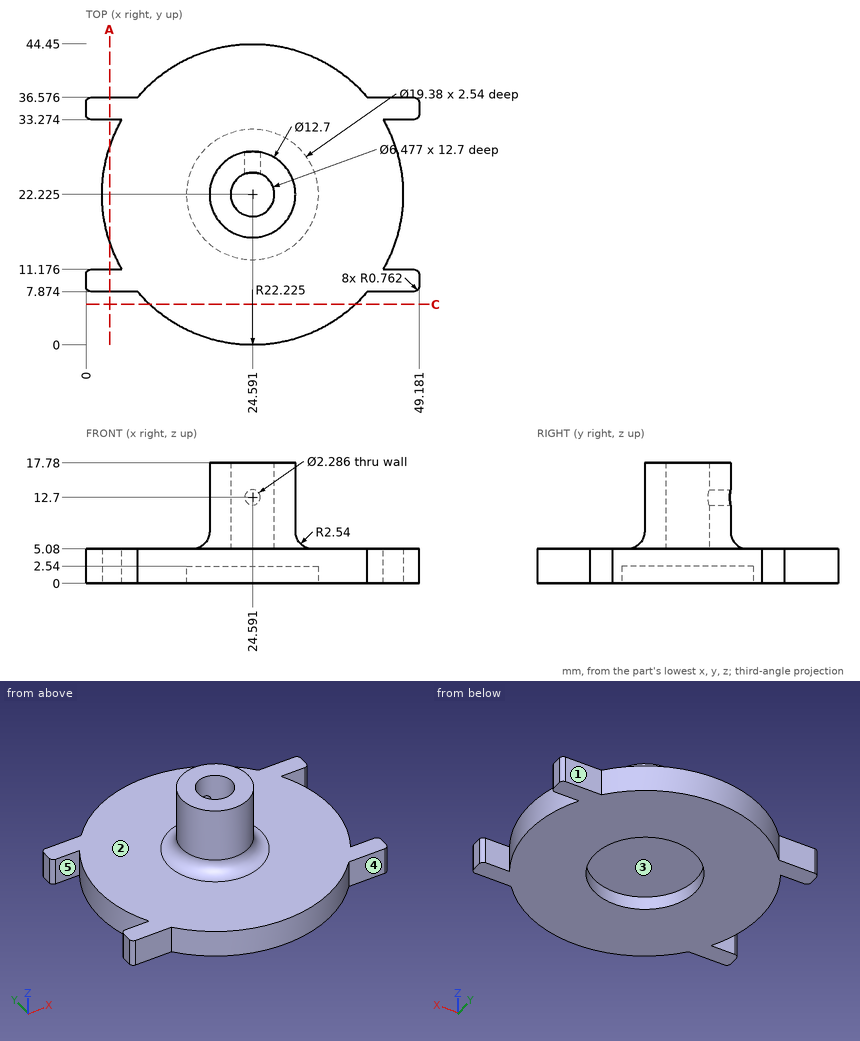
Print and shaded views of the part. All mm, measured from the part's lowest x, y and z. A direction names the side the tool comes from. Give positions to 0.01 mm unless a question says otherwise; leave off trailing zeros. Write each loop counter-clockwise with the first axis right and the second up, starting at its lowest first coordinate (ties: lowest second). Pieces come first, ordered by that corner, then holes. Notation, with made-up numbers: (63.5, 35.5) -> (110.5, 35.5) arc R35 cw to (110.5, 70.5) -> close; hole circle Ø1 at (41.5, 55.5). An arc over 180 degrees is marked (long way). Use CSV: the item, a comma, the result in double quotes. Start each with the question number.
1) Drill centre lines: L1, parallel to Z at x = 13, y = 14; L2, parallel to Y at x = 26.5, z = 7.5 (1 decimal); L3, parallel to X at y = 25, z = 12.75 (1 decimal). Where is each one in solid material? Low to high.
2) Cut at C-C on y = 6. List the corners of the cut face in (x, z).
3) Cut at A-A on x = 3.5. List the corners of the cut face in (y, z) (1 decimal), plus the area to 3 significant figures.
4) Tool access for the marked faces 1, 2, 3, 4 and 5: list every direction of +Z, -Z, +X, -X, +Y, -Y with a clear straight run to the whole face (end or side of a thin tool).
5) Pin check, flat tips, straight feed: P1, Ø5.5, axis at x = 43.5, z = 3, coming from the +Y side (1 decimal); P2, Ø3, axis at x = 25.5, y = 21.5, coming from the +Z side; P3, Ø2.5, axis at x = 3, z = 3.5, coming from the +Y side; P4, Ø10, axis at y = 8, z = 14.5, coming from the +X side. Stop position of each tip, or through.
Final values:
1,L1,"z = 0 to 5.08"
1,L2,"y = 16.2 to 19.6, 24.8 to 28.3"
1,L3,"x = 18.9 to 22.9, 26.3 to 30.3"
2,outline,"(9.4, 0) -> (39.78, 0) -> (39.78, 5.08) -> (9.4, 5.08) -> close"
3,outline,"(7.9, 0) -> (11.2, 0) -> (11.2, 5.1) -> (7.9, 5.1) -> close; (15.2, 0) -> (29.2, 0) -> (29.2, 5.1) -> (15.2, 5.1) -> close; (33.3, 0) -> (36.6, 0) -> (36.6, 5.1) -> (33.3, 5.1) -> close"
3,area,"105 mm2"
4,face 1,"+Z, -Z, +X, +Y"
4,face 2,"+Z"
4,face 3,"-Z"
4,face 4,"+Z, -Z, +X, -Y"
4,face 5,"+Z, -Z, -X"
5,P1,"stops at y = 37.5"
5,P2,"stops at z = 5.08"
5,P3,"stops at y = 36.58"
5,P4,"passes through"
